Here's the drawing with two shaded views (mm, measured from the low corner). I have some questions. Round coordinates to 2 decimals unless told otherwise and drop trailing zeros. Loops run counter-clockwise (first coordinate to the right, second up) from the corner with the lowest first, then second, coordinate; pieces in that order, holes last. Notation, with made-up numbers: (65, -10.75) -> (104, -10.75) arc R26 ccw to (104, 25.25) -> close; hole circle Ø3 at (0, 27). An arc over 180 degrees is marked (long way). Use a Markdown table: item, result.
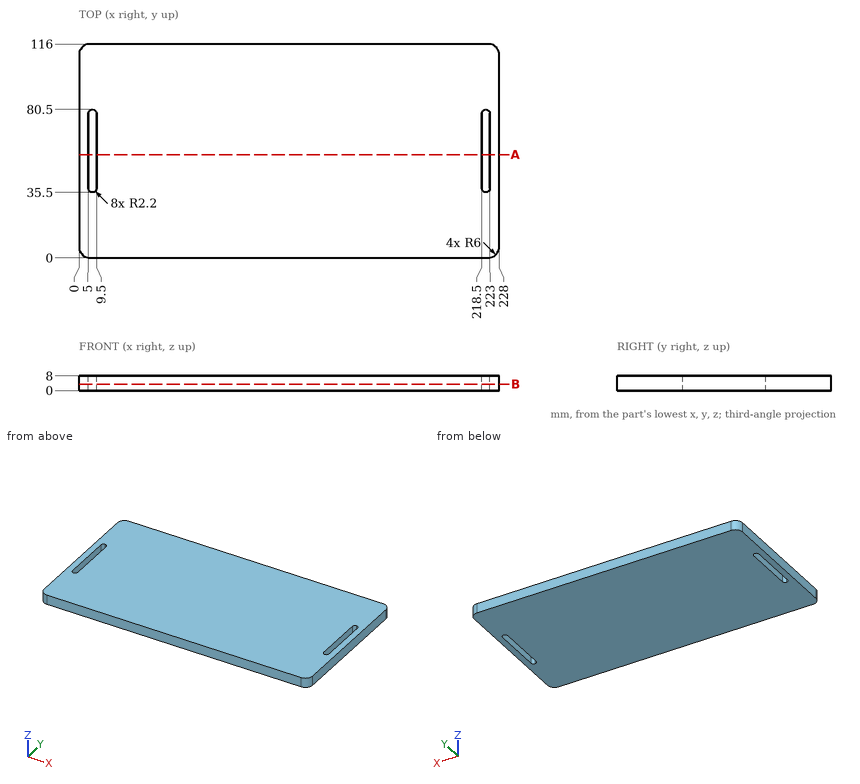
1. I want a section at A-A (y = 56). Please give me the cut outline in (x, z).
Answer sheet:
| item | result |
|---|---|
| outline | (0, 0) -> (5, 0) -> (5, 8) -> (0, 8) -> close; (9.5, 0) -> (218.5, 0) -> (218.5, 8) -> (9.5, 8) -> close; (223, 0) -> (228, 0) -> (228, 8) -> (223, 8) -> close |
2. I want a section at B-B (z = 3.5). Please give me the cut outline in (x, y), plus the area to 3 significant figures.
Answer sheet:
| item | result |
|---|---|
| outline | (0, 6) arc R6 ccw to (6, 0) -> (222, 0) arc R6 ccw to (228, 6) -> (228, 110) arc R6 ccw to (222, 116) -> (6, 116) arc R6 ccw to (0, 110) -> close; hole (5, 37.7) arc R2.2 ccw to (7.2, 35.5) -> (7.3, 35.5) arc R2.2 ccw to (9.5, 37.7) -> (9.5, 78.3) arc R2.2 ccw to (7.3, 80.5) -> (7.2, 80.5) arc R2.2 ccw to (5, 78.3) -> close; hole (218.5, 37.7) arc R2.2 ccw to (220.7, 35.5) -> (220.8, 35.5) arc R2.2 ccw to (223, 37.7) -> (223, 78.3) arc R2.2 ccw to (220.8, 80.5) -> (220.7, 80.5) arc R2.2 ccw to (218.5, 78.3) -> close |
| area | 26,000 mm² |
3. I need wall thicknesses on line 1 (X direction, y = 69.5, z = 3.75); line 2 (X direction, y = 37, z = 6.75); line 3 (X direction, y = 111.5, z = 1.25). Which ranges of each line are inside material? Lowest first, please.
Answer sheet:
| item | result |
|---|---|
| line 1 | x = 0 to 5, 9.5 to 218.5, 223 to 228 |
| line 2 | x = 0 to 5.11, 9.39 to 218.61, 222.89 to 228 |
| line 3 | x = 0.19 to 227.81 |
